The listing builds one solid part. Answer for the finished solid, in the listing's coordinates (mm). Give positions to 0.01 mm unless a question says otherwise; leave off trailing zeros. Loops run counter-clockwise (first coordinate to the right, second up) from the corner with the lowest first, then second, coordinate; pieces in that order, holes last. Notation, with made-up numbers: M 89,67 L 106,67 A19 cw 106,76 Z; hole C -31.75,85.5 d11. An arc over 180 degrees is marked long. Return JSON: item names as keys, results as strings.
from build123d import *

# Parameters (mm, degrees)
SKETCH1_W           = 64.6
SKETCH1_H           = 40.5
SKETCH1_R           = 7.8
SKETCH1_R_2         = 2.2
SKETCH1_R_3         = 1.4
BOSS_EXTRUDE3_DEPTH = 4
SKETCH6_R           = 1.15
CUT_EXTRUDE4_DEPTH  = 5
FILLET4_R           = 0.25


with BuildPart() as part:
    # Sketch1 → Boss-Extrude3 (new body)
    with BuildSketch(Plane(origin=(0, 0, 0), x_dir=(1, 0, 0), z_dir=(0, 1, 0))):
        Rectangle(SKETCH1_W, SKETCH1_H)
        with Locations(Location((9.6, 6.75, 0), (0, 0, 270))):
            Circle(SKETCH1_R, mode=Mode.SUBTRACT)
        with Locations(Location((9.6, -9.25, 0), (0, 0, 270))):
            Circle(SKETCH1_R_2, mode=Mode.SUBTRACT)
        with Locations(Location((-12.25, -8.55, 0), (0, 0, 270))):
            Circle(SKETCH1_R_3, mode=Mode.SUBTRACT)
        with Locations(Location((-8.85, -8.55, 0), (0, 0, 270))):
            Circle(SKETCH1_R_3, mode=Mode.SUBTRACT)
        with Locations(Location((-15.65, -8.55, 0), (0, 0, 270))):
            Circle(SKETCH1_R_3, mode=Mode.SUBTRACT)
    extrude(amount=BOSS_EXTRUDE3_DEPTH)

    # Sketch6 → Cut-Extrude4 (cut)
    with BuildSketch(Plane(origin=(0, 4, 0), x_dir=(1, 0, 0), z_dir=(0, 1, 0))):
        with Locations(Location((-28.2, 16.15, 0), (0, 0, 270))):
            Circle(SKETCH6_R)
        with Locations(Location((28.2, 16.15, 0), (0, 0, 270))):
            Circle(SKETCH6_R)
        with Locations(Location((28.2, -16.15, 0), (0, 0, 270))):
            Circle(SKETCH6_R)
        with Locations(Location((-28.2, -16.15, 0), (0, 0, 270))):
            Circle(SKETCH6_R)
    extrude(amount=-CUT_EXTRUDE4_DEPTH, mode=Mode.SUBTRACT)

    # Fillet4
    fillet4_edges = [part.edges().sort_by_distance(p)[0] for p in [
        (0, 4, 20.25),
        (32.3, 4, 0),
        (0, 4, -20.25),
        (-32.3, 4, 0),
    ]]
    fillet(fillet4_edges, radius=FILLET4_R)


solid = part.part
(1) Straight lines are drawn through the part: line 1 along X through (y, z) = (0.95, 16.15); line 2 along X through (y, z) = (1.15, -17); line 3 along X through (y, z) = (1.25, 8.55). For each, find the intervals that lie inside material, in ascending order.
Values follow:
{"line 1": "-32.3 to -29.35, -27.05 to 27.05, 29.35 to 32.3", "line 2": "-32.3 to -28.97, -27.43 to 27.43, 28.97 to 32.3", "line 3": "-32.3 to -17.05, -14.25 to -13.65, -10.85 to -10.25, -7.45 to 7.51, 11.69 to 32.3"}
(2) Given pin 1 (3.5 mm diameter, centred on x = 9.6, z = 9.25, fed in from -Y), flat-ended and moving along its own axis, determine where the tip first touches the part or whether it passes through.
Values follow:
{"pin 1": "through"}
(3) Determine the mould class of faces 1 (the flat face through (0, 2, -20.25)), 2 (the flat face through (0, 4, 0)), 3 (the cylindrical face through (-27.855, 2.028, 17.247)) for opening direction Z: released by +Z, released by -Z, zero draft, split by the parting line, or undercut.
Values follow:
{"face 1": "released by -Z", "face 2": "zero draft", "face 3": "undercut"}
(4) The part is cut by section D-D (z = 16). Determine the outline of the cut face in (x, y), and give its area (3 significant figures).
Values follow:
{"outline": "M -32.3,0 L -29.34,0 L -29.34,4 L -32.05,4 A0.25 ccw -32.3,3.75 Z; M -27.06,0 L 27.06,0 L 27.06,4 L -27.06,4 Z; M 29.34,0 L 32.3,0 L 32.3,3.75 A0.25 ccw 32.05,4 L 29.34,4 Z", "area": "240 mm²"}
(5) The part is cut by section A-A (x = -12.25). Determine the outline of the cut face in (y, z).
Values follow:
{"outline": "M 0,-20.25 L 3.75,-20.25 A0.25 ccw 4,-20 L 4,7.15 L 0,7.15 Z; M 0,9.95 L 4,9.95 L 4,20 A0.25 ccw 3.75,20.25 L 0,20.25 Z"}
(6) The part is cut by section B-B (y = 0.7). Give the number of separate pieces and of enclosed holes in the cut face, and give its area (3 significant figures).
Values follow:
{"separate pieces": "1", "enclosed holes": "9", "area": "2,370 mm²"}
(7) The part is cut by section C-C (z = -6.75). Determine the outline of the cut face in (x, y).
Values follow:
{"outline": "M -32.3,0 L 1.8,0 L 1.8,4 L -32.05,4 A0.25 ccw -32.3,3.75 Z; M 17.4,0 L 32.3,0 L 32.3,3.75 A0.25 ccw 32.05,4 L 17.4,4 Z"}
